Input: part model. Units: mm. Frame: model coordinates. A direction names the side the tool comes from. Give positions to 0.01 mm unless a question says otherwise; leave off trailing zeros. Loops run counter-clockwise (first coordinate to the right, second up) from the corner with the lowest first, then second, coordinate; pieces in that order, holes last. Notation, with made-up numbers: (80.25, 71.5) - (116.25, 71.5) arc R25 ccw to (116.25, 104.5) - close; hole circle Ø4 at (11.25, 28.25). An arc over 180 degrees is marked (long way). One line per question, with ' | ' between items. Start each with the question number.
Autodesk Inventor part; units mm, degrees
ref_plane "YZ Plane" through (0, 0, 0) normal (1, 0, 0) x (0, 1, 0)
ref_plane "XZ Plane" through (0, 0, 0) normal (0, 1, 0) x (-1, 0, 0)
ref_plane "XY Plane" through (0, 0, 0) normal (0, 0, 1) x (1, 0, 0)
sketch "草圖1" plane through (0, 0, 0) normal (0, 1, 0) x (-1, 0, 0)
  line L0 (0, 0) -> (-40, 0)
  line L1 (-40, 0) -> (-40, 40)
  line L2 (-40, 40) -> (0, 40)
  line L3 (0, 40) -> (0, 0)
  line L4 (-30, 0) -> (-30, 20)
  line L5 (-30, 20) -> (-40, 20)
  line L6 (-30, 40) -> (-40, 30)
  dimension "d0" = 40
  dimension "d1" = 40
  dimension "d2" = 10
  dimension "d3" = 20
  dimension "d4" = 10
  dimension "d5" = 10
extrude "擠出1" add sketch "草圖1" along normal blind 10 contours L0 L4 L5 L1 L6 L2 L3
sketch "草圖2" plane through (0, 0, 0) normal (-1, 0, 0) x (0, 0, 1)
  line L0 (40, 10) -> (40, 0)
  line L1 (40, 0) -> (0, 0)
  line L2 (0, 0) -> (0, 10)
  line L3 (0, 10) -> (40, 10)
  line L4 (40, 10) -> (40, 20)
  line L5 (40, 20) -> (30, 30)
  line L6 (30, 30) -> (10, 30)
  line L7 (10, 30) -> (10, 10)
  line L8 (10, 10) -> (40, 10)
  dimension "d8" = 30
  dimension "d9" = 10
  dimension "d10" = 10
  dimension "d11" = 30
extrude "擠出2" add sketch "草圖2" against normal blind 10 contours L3 L7 L6 L5 L4
equation "\"d10\" = d9"
properties part number "10" material "鋼、碳鋼"
Q1. Section B-B, the plane y = 2.75. Output: boundary loops of the cut face in (x, z), plus the area to 3 significant figures.
Q2. Section A-A, the plane z = 16. Output: boundary loops of the cut face in (x, y).
Q3. Draft query along X for faces 1 (the face through (5, 30, 20)), 2 (the face through (40, 5, 25)), 3 (the face through (0, 15, 20)). Return one class per face: +X half, -X half, draft (parallel to the pull), parting line (faces both ways), or undercut.
Q4. First-contact query: pin 1 (12 mm diameter, centred on x = 35, y = 21.5, fed in from -Z); pin 2 (1.5 mm diameter, centred on x = 6, z = 7, fed in from -Y); pin 3 (20 mm diameter, centred on x = 22.5, z = 21, fed in from +Y); pin 4 (3 mm diameter, centred on x = 6, y = 22.5, fed in from -Z). Flat tips, straight axial feed; report the tip coordinate or a pass-through.
Q5. Line query: L1, parallel to X at y = 7.75, z = 12.5; L2, parallel to X at y = 16, z = 17.5. Output: solid intervals per line, ascending. Write a range as from..to.
Q6. Access query for faces 4 (the face through (35, 5, 35)), 5 (the face through (12, 8, 40)), 6 (the face through (35, 5, 20)), 7 (the face through (5, 20, 10)), 8 (the face through (10, 20, 25)). Directions: +Z, -Z, +X, -X, +Y, -Y. A direction counts if a zero-diameter tool reaches every point of the face in a straight line with its end or side. Return the directions, or none.
Q7. Section C-C, the plane x = 9. Output: boundary loops of the cut face in (y, z), plus the area to 3 significant figures.
Q8. Section D-D, the plane y = 24.75. Output: boundary loops of the cut face in (x, z), plus the area to 4 significant figures.
Solved:
1) outline: (0, 0) - (30, 0) - (30, 20) - (40, 20) - (40, 30) - (30, 40) - (0, 40) - close | area: 1,350 mm²
2) outline: (0, 0) - (30, 0) - (30, 10) - (10, 10) - (10, 30) - (0, 30) - close
3) face 1: draft | face 2: +X half | face 3: -X half
4) pin 1: passes through | pin 2: stops at y = 0 | pin 3: stops at y = 10 | pin 4: stops at z = 10
5) L1: x = 0..30 | L2: x = 0..10
6) face 4: +Z, +X, +Y, -Y | face 5: +Z, +X, -X, +Y, -Y | face 6: -Z, +X, +Y, -Y | face 7: -Z, +X, -X, +Y | face 8: +Z, -Z, +X, +Y
7) outline: (0, 0) - (10, 0) - (10, 10) - (30, 10) - (30, 30) - (20, 40) - (0, 40) - close | area: 950 mm²
8) outline: (0, 10) - (10, 10) - (10, 35.25) - (0, 35.25) - close | area: 252.5 mm²
